Could you check a few things on this model? Use its own coordinates, in mm. A direction names the side the tool comes from. Coordinates: 2 decimals unless noted, no trailing zeros. Loops run counter-clockwise (first coordinate to the right, second up) from the corner with the lowest first, then second, coordinate; pieces in that order, holes last. Notation, with made-up numbers: (-0.75, 23.5) - (16.25, 23.5) arc R15 cw to (16.25, 48.5) - close; hole circle Ø9 at (-34.5, -9.5). An arc over 180 degrees is marked (long way). Use CSV: the item, a comma, the result in double quotes.
Autodesk Fusion 360 part; units mm, degrees
sketch "Sketch1" plane through (0, 0, 0) normal (0, 1, 0) x (1, 0, 0)
  circle A0 centre (0, 0) radius 15
  circle A1 centre (0, 0) radius 25
  line L0 (0, 0) -> (0, -54.75) construction
  circle A2 centre (0, -54.75) radius 2.435
  line L1 (4.5611, -54.75) -> (2.2805, -50.8)
  line L2 (2.2805, -50.8) -> (-2.2805, -50.8)
  line L3 (-2.2805, -50.8) -> (-4.5611, -54.75)
  line L4 (-4.5611, -54.75) -> (-2.2805, -58.7)
  line L5 (-2.2805, -58.7) -> (2.2805, -58.7)
  line L6 (2.2805, -58.7) -> (4.5611, -54.75)
  line L7 (-10, -22.9129) -> (-10, -54.75)
  arc A3 (-10, -54.75) -> (10, -54.75) centre (0, -54.75) ccw
  line L8 (10, -54.75) -> (10, -22.9129)
  line L9 (0, 0) -> (47.4149, 27.375) construction
  line L10 (45.1344, 31.325) -> (42.8538, 27.375)
  circle A4 centre (47.4149, 27.375) radius 2.435
  line L11 (51.976, 27.375) -> (49.6954, 31.325)
  line L12 (42.8538, 27.375) -> (45.1344, 23.425)
  line L13 (49.6954, 23.425) -> (51.976, 27.375)
  line L14 (45.1344, 23.425) -> (49.6954, 23.425)
  arc A5 (52.4149, 18.7147) -> (42.4149, 36.0353) centre (47.4149, 27.375) ccw
  line L15 (49.6954, 31.325) -> (45.1344, 31.325)
  line L16 (42.4149, 36.0353) -> (14.8431, 20.1167)
  line L17 (24.8431, 2.7962) -> (52.4149, 18.7147)
  line L18 (0, 0) -> (-47.4149, 27.375) construction
  line L19 (-49.6954, 23.425) -> (-45.1344, 23.425)
  circle A6 centre (-47.4149, 27.375) radius 2.435
  line L20 (-49.6954, 31.325) -> (-51.976, 27.375)
  line L21 (-45.1344, 23.425) -> (-42.8538, 27.375)
  line L22 (-45.1344, 31.325) -> (-49.6954, 31.325)
  line L23 (-42.8538, 27.375) -> (-45.1344, 31.325)
  arc A7 (-42.4149, 36.0353) -> (-52.4149, 18.7147) centre (-47.4149, 27.375) ccw
  line L24 (-51.976, 27.375) -> (-49.6954, 23.425)
  line L25 (-52.4149, 18.7147) -> (-24.8431, 2.7962)
  line L26 (-14.8431, 20.1167) -> (-42.4149, 36.0353)
  point P0 (0, -54.75)
  point P1 (47.4149, 27.375)
  point P2 (-47.4149, 27.375)
  dimension "d1" = 30
  dimension "d2" = 50
  dimension "d3" = 7.9
  dimension "d4" = 4.87
  dimension "d5" = 50.8
  dimension "d6" = 10
  dimension "d8" = 360
extrude "Extrude1" add sketch "Sketch1" along normal blind 2 contours A1 | A1 A5 L16 L17 | A1 L7 A3 L8 | A1 A7 L25 L26 | L1 L2 L3 L4 L5 L6 | L10 L11 L12 L13 L14 L15 | L19 L20 L21 L22 L23 L24
sketch "Sketch2" plane through (0, 0, 0) normal (0, -1, 0) x (1, 0, 0)
  circle A0 centre (0, 0) radius 15
  circle A1 centre (47.4149, -27.375) radius 2.435
  circle A2 centre (0, 54.75) radius 2.435
  circle A3 centre (-47.4149, -27.375) radius 2.435
  line L0 (-42.4149, -36.0353) -> (-14.8431, -20.1167)
  arc A4 (-14.8431, -20.1167) -> (14.8431, -20.1167) centre (0, 0) ccw
  line L1 (14.8431, -20.1167) -> (42.4149, -36.0353)
  arc A5 (42.4149, -36.0353) -> (52.4149, -18.7147) centre (47.4149, -27.375) ccw
  line L2 (52.4149, -18.7147) -> (24.8431, -2.7962)
  arc A6 (24.8431, -2.7962) -> (10, 22.9129) centre (0, 0) ccw
  line L3 (10, 22.9129) -> (10, 54.75)
  arc A7 (10, 54.75) -> (-10, 54.75) centre (0, 54.75) ccw
  line L4 (-10, 54.75) -> (-10, 22.9129)
  arc A8 (-10, 22.9129) -> (-24.8431, -2.7962) centre (0, 0) ccw
  line L5 (-24.8431, -2.7962) -> (-52.4149, -18.7147)
  arc A9 (-52.4149, -18.7147) -> (-42.4149, -36.0353) centre (-47.4149, -27.375) ccw
  line L6 (2.2372, 50.875) -> (4.4745, 54.75)
  line L7 (4.4745, 54.75) -> (2.2372, 58.625)
  line L8 (2.2372, 58.625) -> (-2.2372, 58.625)
  line L9 (-2.2372, 58.625) -> (-4.4745, 54.75)
  line L10 (-4.4745, 54.75) -> (-2.2372, 50.875)
  line L11 (-2.2372, 50.875) -> (2.2372, 50.875)
  line L12 (-51.8894, -27.375) -> (-49.6521, -31.25)
  line L13 (-45.1777, -23.5) -> (-49.6521, -23.5)
  line L14 (-42.9404, -27.375) -> (-45.1777, -23.5)
  line L15 (-49.6521, -31.25) -> (-45.1777, -31.25)
  circle A10 centre (-47.4149, -27.375) radius 2.435
  line L16 (-45.1777, -31.25) -> (-42.9404, -27.375)
  line L17 (-49.6521, -23.5) -> (-51.8894, -27.375)
  line L18 (49.6521, -31.25) -> (51.8894, -27.375)
  line L19 (42.9404, -27.375) -> (45.1777, -31.25)
  line L20 (45.1777, -23.5) -> (42.9404, -27.375)
  line L21 (51.8894, -27.375) -> (49.6521, -23.5)
  circle A11 centre (47.4149, -27.375) radius 2.435
  line L22 (49.6521, -23.5) -> (45.1777, -23.5)
  line L23 (45.1777, -31.25) -> (49.6521, -31.25)
  point P0 (0, 54.75)
  point P1 (-47.4149, -27.375)
  point P2 (47.4149, -27.375)
  dimension "d11" = 7.75
  dimension "d13" = 360
extrude "Extrude2" add sketch "Sketch2" along normal blind 7 contours L6 L7 L8 L9 L10 L11 | L12 L13 L14 L15 L16 L17 | L18 L19 L20 L21 L22 L23
sketch "Sketch3" plane through (0, 2, 0) normal (0, 1, 0) x (-1, 0, 0)
  circle A0 centre (0, 0) radius 15
  circle A1 centre (-47.4149, -27.375) radius 2.435
  circle A2 centre (0, 54.75) radius 2.435
  circle A3 centre (47.4149, -27.375) radius 2.435
  line L0 (14.8431, -20.1167) -> (42.4149, -36.0353)
  arc A4 (42.4149, -36.0353) -> (52.4149, -18.7147) centre (47.4149, -27.375) ccw
  line L1 (52.4149, -18.7147) -> (24.8431, -2.7962)
  arc A5 (24.8431, -2.7962) -> (10, 22.9129) centre (0, 0) ccw
  line L2 (10, 22.9129) -> (10, 54.75)
  arc A6 (10, 54.75) -> (-10, 54.75) centre (0, 54.75) ccw
  line L3 (-10, 54.75) -> (-10, 22.9129)
  arc A7 (-10, 22.9129) -> (-24.8431, -2.7962) centre (0, 0) ccw
  line L4 (-24.8431, -2.7962) -> (-52.4149, -18.7147)
  arc A8 (-52.4149, -18.7147) -> (-42.4149, -36.0353) centre (-47.4149, -27.375) ccw
  line L5 (-42.4149, -36.0353) -> (-14.8431, -20.1167)
  arc A9 (-14.8431, -20.1167) -> (14.8431, -20.1167) centre (0, 0) ccw
  line L6 (0, 54.75) -> (0, 15) construction
  circle A10 centre (0, 23) radius 3
  circle A11 centre (0, 23) radius 1.575
  circle A12 centre (-19.9186, -11.5) radius 3
  circle A13 centre (-19.9186, -11.5) radius 1.575
  circle A14 centre (19.9186, -11.5) radius 3
  circle A15 centre (19.9186, -11.5) radius 1.575
  dimension "d16" = 8
  dimension "d17" = 6
  dimension "d18" = 3.15
  dimension "d20" = 360
extrude "Extrude6" cut sketch "Sketch3" against normal up to surface (2 mm away) contours A11 | A13 | A15
sketch "Sketch5" plane through (0, 0, 0) normal (0, -1, 0) x (1, 0, 0)
  circle A0 centre (19.9186, -11.5) radius 1.575
  circle A1 centre (0, 23) radius 1.575
  circle A2 centre (-19.9186, -11.5) radius 1.575
  line L0 (-2.2372, 50.875) -> (-4.4745, 54.75)
  line L1 (-4.4745, 54.75) -> (-2.2372, 58.625)
  line L2 (-2.2372, 58.625) -> (2.2372, 58.625)
  line L3 (2.2372, 58.625) -> (4.4745, 54.75)
  line L4 (4.4745, 54.75) -> (2.2372, 50.875)
  line L5 (2.2372, 50.875) -> (-2.2372, 50.875)
  line L6 (-49.6521, -23.5) -> (-45.1777, -23.5)
  line L7 (-45.1777, -23.5) -> (-42.9404, -27.375)
  line L8 (-42.9404, -27.375) -> (-45.1777, -31.25)
  line L9 (-45.1777, -31.25) -> (-49.6521, -31.25)
  line L10 (-49.6521, -31.25) -> (-51.8894, -27.375)
  line L11 (-51.8894, -27.375) -> (-49.6521, -23.5)
  line L12 (45.1777, -31.25) -> (42.9404, -27.375)
  line L13 (42.9404, -27.375) -> (45.1777, -23.5)
  line L14 (45.1777, -23.5) -> (49.6521, -23.5)
  line L15 (49.6521, -23.5) -> (51.8894, -27.375)
  line L16 (51.8894, -27.375) -> (49.6521, -31.25)
  line L17 (49.6521, -31.25) -> (45.1777, -31.25)
  circle A3 centre (0, 0) radius 15
  line L18 (-42.4149, -36.0353) -> (-14.8431, -20.1167)
  arc A4 (-14.8431, -20.1167) -> (14.8431, -20.1167) centre (0, 0) ccw
  line L19 (14.8431, -20.1167) -> (42.4149, -36.0353)
  arc A5 (42.4149, -36.0353) -> (52.4149, -18.7147) centre (47.4149, -27.375) ccw
  line L20 (52.4149, -18.7147) -> (24.8431, -2.7962)
  arc A6 (24.8431, -2.7962) -> (10, 22.9129) centre (0, 0) ccw
  line L21 (10, 22.9129) -> (10, 54.75)
  arc A7 (10, 54.75) -> (-10, 54.75) centre (0, 54.75) ccw
  line L22 (-10, 54.75) -> (-10, 22.9129)
  arc A8 (-10, 22.9129) -> (-24.8431, -2.7962) centre (0, 0) ccw
  line L23 (-24.8431, -2.7962) -> (-52.4149, -18.7147)
  arc A9 (-52.4149, -18.7147) -> (-42.4149, -36.0353) centre (-47.4149, -27.375) ccw
  line L24 (2.2372, 26.875) -> (-2.2372, 26.875)
  line L25 (-2.2372, 26.875) -> (-4.4745, 23)
  line L26 (-4.4745, 23) -> (-2.2372, 19.125)
  line L27 (-2.2372, 19.125) -> (2.2372, 19.125)
  line L28 (2.2372, 19.125) -> (4.4745, 23)
  line L29 (4.4745, 23) -> (2.2372, 26.875)
  line L30 (-22.1558, -15.375) -> (-17.6814, -15.375)
  line L31 (-22.1558, -7.625) -> (-24.393, -11.5)
  circle A10 centre (-19.9186, -11.5) radius 1.575
  line L32 (-17.6814, -15.375) -> (-15.4441, -11.5)
  line L33 (-24.393, -11.5) -> (-22.1558, -15.375)
  line L34 (-15.4441, -11.5) -> (-17.6814, -7.625)
  line L35 (-17.6814, -7.625) -> (-22.1558, -7.625)
  line L36 (24.393, -11.5) -> (22.1558, -7.625)
  line L37 (17.6814, -15.375) -> (22.1558, -15.375)
  circle A11 centre (19.9186, -11.5) radius 1.575
  line L38 (22.1558, -7.625) -> (17.6814, -7.625)
  line L39 (22.1558, -15.375) -> (24.393, -11.5)
  line L40 (17.6814, -7.625) -> (15.4441, -11.5)
  line L41 (15.4441, -11.5) -> (17.6814, -15.375)
  point P0 (0, 23)
  point P1 (-19.9186, -11.5)
  point P2 (19.9186, -11.5)
  dimension "d32" = 7.75
  dimension "d34" = 360
extrude "Extrude7" cut sketch "Sketch5" against normal up to surface (1 mm away) contours L24 L25 L26 L27 L28 L29 | L30 L31 L32 L33 L34 L35 | L36 L37 L38 L39 L40 L41
(1) Thinking about a two-plate mould opening in Z: for faces 1 (the face through (-18.7, 1.5, -12.5)), 2 (the face through (28.822, 0.986, -28.187)), 3 (the face through (55.963, 0.986, -32.564)), which applies, +Z half, -Z half, draft (parallel to the pull), parting line (faces both ways), or undercut?
Computed:
face 1,"undercut"
face 2,"-Z half"
face 3,"parting line"
(2) Please list where these lines run through material, in increasing order: line 1 (Z direction, x = 0, y = 1.5) (3 decimals); line 2 (Z direction, x = 0, y = -1.5) (3 decimals); line 3 (X direction, y = -3, z = 54.75) (1 decimal).
Computed:
line 1,"z = -25 to -15, 15 to 21.425, 24.575 to 52.315, 57.185 to 64.75"
line 2,"z = 50.875 to 52.315, 57.185 to 58.625"
line 3,"x = -4.5 to -2.4, 2.4 to 4.5"
(3) Will these pins go through, and if not, where does the flat tip stop? pin 1 (1.3 mm diameter, centred on x = -48.5, y = -3.5, fed in from -Z); pin 2 (5 mm diameter, centred on x = -47, y = -3.5, fed in from +Z); pin 3 (0.6 mm diameter, centred on y = 0.5, z = 43.5, fed in from +X).
Computed:
pin 1,"stops at z = -31.25"
pin 2,"stops at z = -23.5"
pin 3,"stops at x = 10"
(4) Suppose I cut it at B-B (z = 0). Write out the boundary of the cut face in (x, y), plus the area to 3 significant figures.
Computed:
outline,"(-25, 0) - (-15, 0) - (-15, 2) - (-25, 2) - close; (15, 0) - (25, 0) - (25, 2) - (15, 2) - close"
area,"40.0 mm²"
(5) Suppose I cut it at A-A (y = -5.5). State how many separate pieces and enclosed holes the cut face has, plus the area to 3 significant figures.
Computed:
separate pieces,"3"
enclosed holes,"3"
area,"100 mm²"
(6) Suppose I cut it at D-D (x = 48). Write out the boundary of the cut face in (y, z), plus the area to 3 significant figures.
Computed:
outline,"(-7, -31.25) - (0, -31.25) - (0, -37.36) - (2, -37.36) - (2, -29.74) - (-7, -29.74) - close; (-7, -25.01) - (2, -25.01) - (2, -16.17) - (0, -16.17) - (0, -23.5) - (-7, -23.5) - close"
area,"54.1 mm²"
(7) Which directions (+Z, -Z, +X, -X, +Y, -Y) give clear straight access to the entire face, cutting with the end or side of a thin tool? Please do faces 4 (the face through (-50.755, -3.451, -25.41)), 5 (the face through (-3.37, -3.45, 52.84)), 6 (the face through (-47, -3, -31.25)), 7 (the face through (47, -3, -23.5)), 8 (the face through (50.755, -3.451, -29.34)).
Computed:
face 4,"+Z, -X, -Y"
face 5,"-Z, -X, -Y"
face 6,"-Z, +X, -X, -Y"
face 7,"+Z, +X, -X, -Y"
face 8,"-Z, +X, -Y"
(8) Suppose I cut it at C-C (x = 0). Write out the boundary of the cut face in (y, z) (3 decimals), plus the area to 3 significant figures.
Computed:
outline,"(-7, 50.875) - (0, 50.875) - (0, 26.875) - (1, 26.875) - (1, 24.575) - (2, 24.575) - (2, 52.315) - (-7, 52.315) - close; (-7, 57.185) - (2, 57.185) - (2, 64.75) - (0, 64.75) - (0, 58.625) - (-7, 58.625) - close; (0, -25) - (2, -25) - (2, -15) - (0, -15) - close; (0, 15) - (2, 15) - (2, 21.425) - (1, 21.425) - (1, 19.125) - (0, 19.125) - close"
area,"119 mm²"
